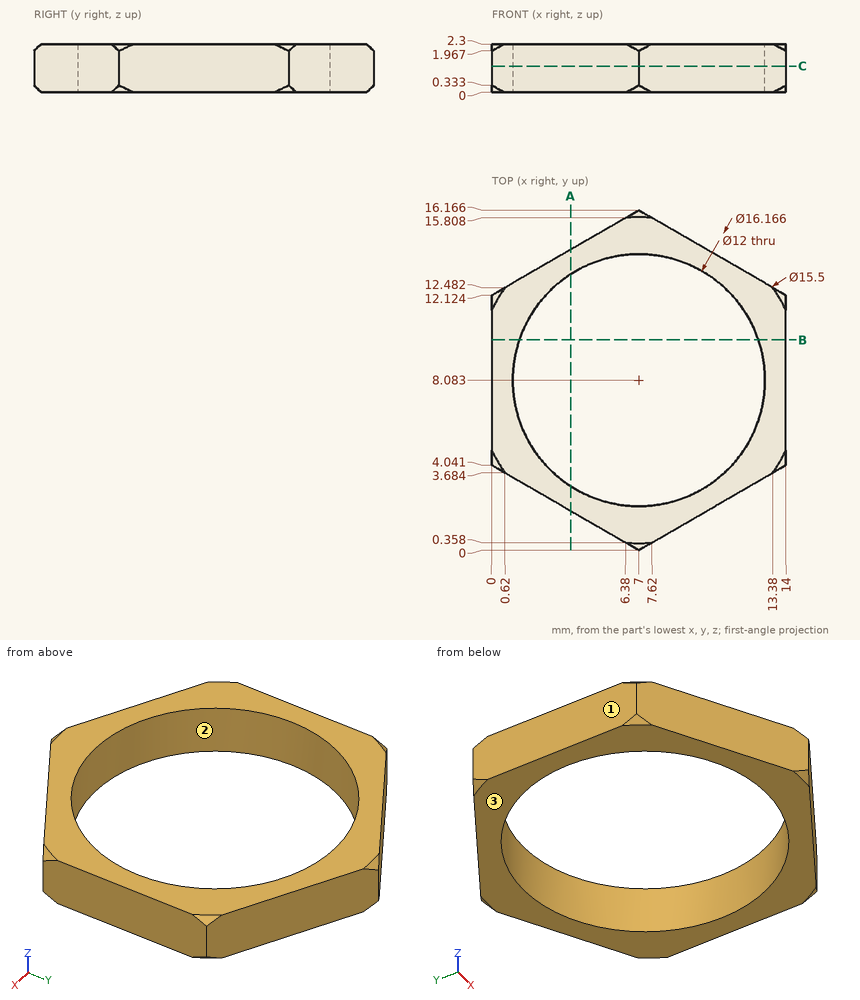
Verification items for this drawing (mm, ordinates from the low corner). Coordinates: 2 decimals unless noted, no trailing zeros. Order: outer loops, then holes, each group sorted by start corner. A loop starts at its lowest first (then second) coordinate and runs counter-clockwise, first axis right, second up. Notation, with made-up numbers: (2, 29) -> (58, 29) arc R14 cw to (58, 33) -> close; hole circle Ø5 at (-9, -18.5). An arc over 180 degrees is marked (long way). Put each result on its own line as item: value. Start each with the question number.
1. Cross-section at A-A, the plane x = 3.75. Record the boundary of the cut face in (y, z).
2. Material ranges on L1, parallel to X at y = 12.5, z = 0.8; L2, parallel to Y at x = 9, z = 1.05 (1 decimal); L3, parallel to Y at x = 4.75, z = 1.05 (1 decimal), recorded low to high. Write a range as [from, to].
3. Cross-section at C-C, the plane z = 1.25. Record the boundary of the cut face in (x, y) (1 decimal).
4. Mould release check, pull along X, two halves, no side actions. Record for the marked faces 1, 2 and 3: released by +X, released by -X, zero draft, split by the parting line, or undercut.
5. Cross-section at B-B, the plane y = 10. Record the boundary of the cut face in (x, z) (1 decimal).
Computed:
1. outline: (1.88, 0) -> (3.04, 0) -> (3.04, 2.3) -> (1.88, 2.3) -> close; (13.13, 0) -> (14.29, 0) -> (14.29, 2.3) -> (13.13, 2.3) -> close
2. L1: [0.65, 2.94], [11.06, 13.35]
2. L2: [1.2, 2.4], [13.7, 15]
2. L3: [1.3, 2.5], [13.6, 14.9]
3. outline: (0, 4) -> (7, 0) -> (14, 4) -> (14, 12.1) -> (7, 16.2) -> (0, 12.1) -> close; hole circle Ø12 at (7, 8.1)
4. face 1: released by -X
4. face 2: undercut
4. face 3: zero draft
5. outline: (0, 0) -> (1.3, 0) -> (1.3, 2.3) -> (0, 2.3) -> close; (12.7, 0) -> (14, 0) -> (14, 2.3) -> (12.7, 2.3) -> close
